from build123d import *

# Parameters (mm, degrees)
SKETCH1_R               = 17.5
SKETCH1_R_2             = 12
BOSS_EXTRUDE1_DEPTH     = 30
BOSS_EXTRUDE2_DEPTH     = 14
CUT_EXTRUDE1_DEPTH      = 10
SKETCH8_W               = 84
SKETCH8_H               = 18
CUT_EXTRUDE2_DEPTH      = 19
SKETCH9_W               = 10
SKETCH9_H               = 18
CUT_EXTRUDE3_DEPTH      = 68
SKETCH10_W              = 12
SKETCH10_H              = 10
CUT_EXTRUDE4_DEPTH      = 43
CUT_EXTRUDE4_DEPTH_BACK = 43
CUT_EXTRUDE5_REACH      = 69
SKETCH7_R               = 4
FILLET2_R               = 1


with BuildPart() as part:
    # Sketch1 → Boss-Extrude1 (new body, symmetric)
    with BuildSketch(Plane(origin=(0, 0, 0), x_dir=(1, 0, 0), z_dir=(0, 1, 0))):
        Circle(SKETCH1_R)
        Circle(SKETCH1_R_2, mode=Mode.SUBTRACT)
    extrude(amount=BOSS_EXTRUDE1_DEPTH, both=True)

    # Sketch5 → Boss-Extrude2 (add, symmetric)
    with BuildSketch(Plane(origin=(0, 0, 0), x_dir=(1, 0, 0), z_dir=(0, 1, 0))):
        Polygon((42, -16), (-42, -16), (-42, -25), (-12, -25), (-12, -22), (12, -22), (12, -25), (42, -25), align=None)
        with BuildLine():
            Line((-25, 42), (-25, -16))
            Line((-25, -16), (-7.088723439, -16))
            ThreePointArc((-7.088723439, -16), (0, 17.5), (7.088723439, -16))
            Line((7.088723439, -16), (25, -16))
            Line((25, -16), (25, 42))
            Line((25, 42), (15, 42))
            ThreePointArc((15, 42), (0, 27), (-15, 42))
            Line((-15, 42), (-25, 42))
        make_face()
    extrude(amount=BOSS_EXTRUDE2_DEPTH, both=True)

    # Sketch6 → Cut-Extrude1 (cut, through all)
    with BuildSketch(Plane(origin=(0, 0, 16), x_dir=(-1, 0, 0), z_dir=(0, 0, -1))):
        with BuildLine():
            Line((35, 6), (49, 6))
            ThreePointArc((49, 6), (55, 0), (49, -6))
            Line((49, -6), (35, -6))
            ThreePointArc((35, -6), (29, 0), (35, 6))
        make_face()
        with BuildLine():
            Line((-35, 6), (-49, 6))
            ThreePointArc((-49, 6), (-55, 0), (-49, -6))
            Line((-49, -6), (-35, -6))
            ThreePointArc((-35, -6), (-29, 0), (-35, 6))
        make_face()
    extrude(amount=-CUT_EXTRUDE1_DEPTH, mode=Mode.SUBTRACT)

    # Sketch8 → Cut-Extrude2 (cut, symmetric)
    with BuildSketch(Plane(origin=(0, 0, 0), x_dir=(0, 0, -1), z_dir=(1, 0, 0))):
        Rectangle(SKETCH8_W, SKETCH8_H)
    extrude(amount=CUT_EXTRUDE2_DEPTH, both=True, mode=Mode.SUBTRACT)

    # Sketch9 → Cut-Extrude3 (cut, through all)
    with BuildSketch(Plane.ZY.offset(25)):
        with Locations((-37, 0)):
            Rectangle(SKETCH9_W, SKETCH9_H)
    extrude(amount=-CUT_EXTRUDE3_DEPTH, mode=Mode.SUBTRACT)

    # Sketch10 → Cut-Extrude4 (cut, two sides)
    with BuildSketch(Plane(origin=(0, 0, 0), x_dir=(0, 0, -1), z_dir=(1, 0, 0))) as cut_extrude4_sk:
        with Locations((0, -25)):
            Rectangle(SKETCH10_W, SKETCH10_H)
        with Locations((0, 25)):
            Rectangle(SKETCH10_W, SKETCH10_H)
    extrude(amount=CUT_EXTRUDE4_DEPTH, mode=Mode.SUBTRACT)
    extrude(cut_extrude4_sk.sketch, amount=-CUT_EXTRUDE4_DEPTH_BACK, mode=Mode.SUBTRACT)

    # Sketch7 → Cut-Extrude5 (cut, up to next)
    with BuildSketch(Plane.ZY.offset(25), mode=Mode.PRIVATE) as cut_extrude5_sk1:
        with Locations((-12, 0)):
            Circle(SKETCH7_R)
    cut_extrude5_tool1 = extrude(cut_extrude5_sk1.sketch, amount=-CUT_EXTRUDE5_REACH, mode=Mode.PRIVATE) & part.part
    add(cut_extrude5_tool1.solids().sort_by_distance((-25, 0, -12))[0], mode=Mode.SUBTRACT)

    # Fillet2
    fillet2_edges = [part.edges().sort_by_distance(p)[0] for p in [
        (-17.5, -14, 0),
        (-17.5, 14, 0),
        (25, 14, -13),
        (-25, 14, -13),
        (-25, -14, -13),
        (25, -14, -13),
    ]]
    fillet(fillet2_edges, radius=FILLET2_R)


solid = part.part
Source: CAD feature listing. Evaluate the final solid. Frame: model axes, mm. A direction names the side the tool comes from. Coordinates: 2 decimals unless noted, no trailing zeros. Loops run counter-clockwise (first coordinate to the right, second up) from the corner with the lowest first, then second, coordinate; pieces in that order, holes last. Notation, with made-up numbers: (67, -39) - (107, -39) arc R18 cw to (107, -31) - close; hole circle Ø3 at (54.5, -22). An arc over 180 degrees is marked (long way). One line per item, written item: value. Start each with the question number.
1. Set-up query: faces 1 (the flat face through (13, 25, 6)), 2 (the flat face through (-39, -6, 20)), 3 (the flat face through (-13, -25, -6)). Return all of +Z, -Z, +X, -X, +Y, -Y with unobstructed straight access to the full face (end or side cutting, diameter ignored); none if empty.
2. Section A-A (x = 0). Return the cut outline in (y, z), and give its area (3 significant figures).
3. Ray query, L1, parallel to Y at x = -21.05, z = -12; L2, parallel to Z at x = 0, y = -23; L3, parallel to X at y = -5, z = -10.5. Return the intervals inside material, ascending.
4. Mould query, pull axis Z, two halves, no side actions, for faces 4 (the flat face through (29, 3, 16)), 5 (the cylindrical face through (8.075, 22.605, 15.526)), 6 (the flat face through (15, 20, 0)), 7 (the flat face through (0, -11, 22)). Classes: pulls with the +Z half, pulls with the -Z half, needs draft (parallel to the pull), parting line crosses it, or undercut.
5. Contact query for flat-ended pins moving along their axis: P1, Ø3, axis at x = -14.5, y = -23, coming from the +Z side; P2, Ø6.5, axis at x = 12.5, y = -26.5, coming from the +Z side; P3, Ø5.5, axis at x = 13, z = 1.5, coming from the -Y side; P4, Ø15, axis at x = 2, z = -18.5, coming from the +Y side. Output: stop coordinate, or through.
6. Section C-C (x = 37). Return the cut outline in (y, z).
7. Section B-B (y = -22.5). Return the cut outline in (x, z), and give its area (3 significant figures).
8. Section D-D (z = -26). Return the cut outline in (x, y).
Verdict:
1. face 1: +X, -X, +Y
1. face 2: +Z, -Z, -X
1. face 3: +X, -X, -Y
2. outline: (-30, -17.5) - (-15, -17.5) arc R1 cw to (-14, -18.5) - (-14, -27) - (-9, -27) - (-9, -12) - (-30, -12) - close; (-30, 12) - (-9, 12) - (-9, 22) - (-14, 22) - (-14, 18.5) arc R1 cw to (-15, 17.5) - (-30, 17.5) - close; (9, -27) - (14, -27) - (14, -18.5) arc R1 cw to (15, -17.5) - (30, -17.5) - (30, -12) - (9, -12) - close; (9, 12) - (30, 12) - (30, 17.5) - (15, 17.5) arc R1 cw to (14, 18.5) - (14, 22) - (9, 22) - close
2. area: 603 mm2
3. L1: y = -14 to -4, 4 to 14
3. L2: z = -17.5 to -12, 12 to 17.5
3. L3: x = -25 to -19, 19 to 25
4. face 4: pulls with the -Z half
4. face 5: parting line crosses it
4. face 6: undercut
4. face 7: pulls with the +Z half
5. P1: stops at z = 11.72
5. P2: stops at z = 14.86
5. P3: stops at y = -20
5. P4: stops at y = 30
6. outline: (-14, 16) - (-6, 16) - (-6, 25) - (-14, 25) - close; (6, 16) - (14, 16) - (14, 25) - (6, 25) - close
7. outline: (-16.44, -6) arc R17.5 ccw to (16.44, -6) - (10.39, -6) arc R12 cw to (-10.39, -6) - close; (-16.44, 6) - (-10.39, 6) arc R12 cw to (10.39, 6) - (16.44, 6) arc R17.5 ccw to start
7. area: 374 mm2
8. outline: (-25, -13) arc R1 ccw to (-24, -14) - (24, -14) arc R1 ccw to (25, -13) - (25, 13) arc R1 ccw to (24, 14) - (-24, 14) arc R1 ccw to (-25, 13) - close; hole (-19, -9) - (19, -9) - (19, 9) - (-19, 9) - close
